from build123d import *

# Parameters (mm, degrees)
SKETCH1_W           = 129.54
SKETCH1_H           = 25.4
BOSS_EXTRUDE1_DEPTH = 6.35
SKETCH2_R           = 3.175
SKETCH2_R_2         = 8.73125
CUT_EXTRUDE1_DEPTH  = 67.30810961
SKETCH3_R           = 10.16
CUT_EXTRUDE2_DEPTH  = 1.27
CUT_EXTRUDE3_DEPTH  = 67.30810961
FILLET1_R           = 1.27


with BuildPart() as part:
    # Sketch1 → Boss-Extrude1 (new body)
    with BuildSketch(Plane(origin=(0, 0, 0), x_dir=(1, 0, 0), z_dir=(0, 1, 0))):
        Rectangle(SKETCH1_W, SKETCH1_H)
    extrude(amount=BOSS_EXTRUDE1_DEPTH)

    # Sketch2 → Cut-Extrude1 (cut, through all)
    with BuildSketch(Plane(origin=(0, 6.35, 0), x_dir=(1, 0, 0), z_dir=(0, 1, 0))):
        with Locations(Location((-52.07, 0, 0), (0, 0, 270))):
            Circle(SKETCH2_R)
        with Locations(Location((26.67, 0, 0), (0, 0, 270))):
            Circle(SKETCH2_R)
        with Locations(Location((52.07, 0, 0), (0, 0, 270))):
            Circle(SKETCH2_R)
        with Locations(Location((-1.27, 0, 0), (0, 0, 270))):
            Circle(SKETCH2_R_2)
    extrude(amount=-CUT_EXTRUDE1_DEPTH, mode=Mode.SUBTRACT)

    # Sketch3 → Cut-Extrude2 (cut)
    with BuildSketch(Plane(origin=(0, 0, 0), x_dir=(-1, 0, 0), z_dir=(0, -1, 0))):
        with Locations(Location((1.27, 0, 0), (0, 0, 90))):
            Circle(SKETCH3_R)
    extrude(amount=-CUT_EXTRUDE2_DEPTH, mode=Mode.SUBTRACT)

    # Sketch5 → Cut-Extrude3 (cut, through all)
    with BuildSketch(Plane(origin=(0, 6.35, 0), x_dir=(1, 0, 0), z_dir=(0, 1, 0))):
        with BuildLine():
            ThreePointArc((-64.77, -3.9e-08), (-61.050256152, 8.98025609), (-52.070000049, 12.7))
            Line((-52.070000049, 12.7), (-64.77, 12.7))
            Line((-64.77, 12.7), (-64.77, -3.9e-08))
        make_face()
        with BuildLine():
            Line((-64.77, -12.7), (-52.07, -12.7))
            ThreePointArc((-52.07, -12.7), (-61.050256107, -8.980256135), (-64.77, -3.9e-08))
            Line((-64.77, -3.9e-08), (-64.77, -12.7))
        make_face()
        with BuildLine():
            ThreePointArc((64.77, 0), (61.050256132, -8.98025611), (52.07000003, -12.7))
            Line((52.07000003, -12.7), (64.77, -12.7))
            Line((64.77, -12.7), (64.77, 0))
        make_face()
        with BuildLine():
            Line((64.77, 12.7), (52.07, 12.7))
            ThreePointArc((52.07, 12.7), (61.050256121, 8.980256121), (64.77, 0))
            Line((64.77, 0), (64.77, 12.7))
        make_face()
    extrude(amount=-CUT_EXTRUDE3_DEPTH, mode=Mode.SUBTRACT)

    # Fillet1
    fillet1_edges = [part.edges().sort_by_distance(p)[0] for p in [
        (-2.4e-08, 0, -12.7),
        (-2.4e-08, 6.35, -12.7),
        (-64.77, 6.35, 2.4e-08),
        (-64.77, 0, 2.4e-08),
        (64.77, 6.35, -1.5e-08),
        (64.77, 0, -1.5e-08),
        (1.5e-08, 0, 12.7),
        (1.5e-08, 6.35, 12.7),
    ]]
    fillet(fillet1_edges, radius=FILLET1_R)


solid = part.part
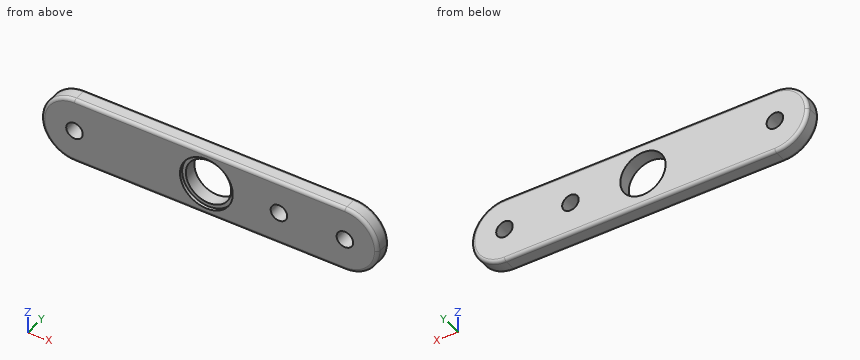
Input: part model. Units: mm. Frame: model coordinates. Round coordinates to 2 decimals unless told otherwise and drop trailing zeros. Write each loop counter-clockwise with the first axis right and the second up, starting at its lowest first coordinate (ties: lowest second). Pieces come first, ordered by that corner, then holes.
1) Contact query for a flat-ended pin moving along its axis: P1, Ø3, axis at y = 5.5, z = 7.5, coming from the +X side. Output: stop coordinate, or through.
2) Cut plane A-A (x = -1.27). Return the cut outline in (y, z).
3) Ray query, L1, parallel to Y at x = 6, z = -5.75; L2, parallel to X at y = 2, z = -6.25; L3, parallel to Z at x = -51, y = 5.25. Return the intervals inside material, ascending.
4) Cut plane B-B (y = 3). Count the separate pieces of the cut face and the enclosed holes in it, then the cut area to 3 significant figures.
5) Cut plane C-C (x = 26.67). Return the cut outline in (y, z) (3 decimals), then the cut area to 3 significant figures.
Geometry says:
1. P1: stops at x = 63.24
2. outline: (0, -11.43) arc R1.27 ccw to (1.27, -12.7) - (5.08, -12.7) arc R1.27 ccw to (6.35, -11.43) - (6.35, -8.73) - (1.27, -8.73) - (1.27, -10.16) - (0, -10.16) - close; (0, 10.16) - (1.27, 10.16) - (1.27, 8.73) - (6.35, 8.73) - (6.35, 11.43) arc R1.27 ccw to (5.08, 12.7) - (1.27, 12.7) arc R1.27 ccw to (0, 11.43) - close
3. L1: y = 1.27 to 6.35
3. L2: x = -63.13 to -7.37, 4.83 to 63.13
3. L3: z = -12.69 to -2.99, 2.99 to 12.69
4. separate pieces: 1
4. enclosed holes: 4
4. area: 2,820 mm2
5. outline: (0, -11.43) arc R1.27 ccw to (1.27, -12.7) - (5.08, -12.7) arc R1.27 ccw to (6.35, -11.43) - (6.35, -3.175) - (0, -3.175) - close; (0, 3.175) - (6.35, 3.175) - (6.35, 11.43) arc R1.27 ccw to (5.08, 12.7) - (1.27, 12.7) arc R1.27 ccw to (0, 11.43) - close
5. area: 120 mm2
